CAD build for the part. Positions are in the model's coordinates, mm. Face numbers are marked on the shaded views. Coordinates: 2 decimals unless noted, no trailing zeros. Write each loop counter-clockwise with the first axis right and the second up, starting at its lowest first coordinate (ties: lowest second). Pieces come first, ordered by that corner, then holes.
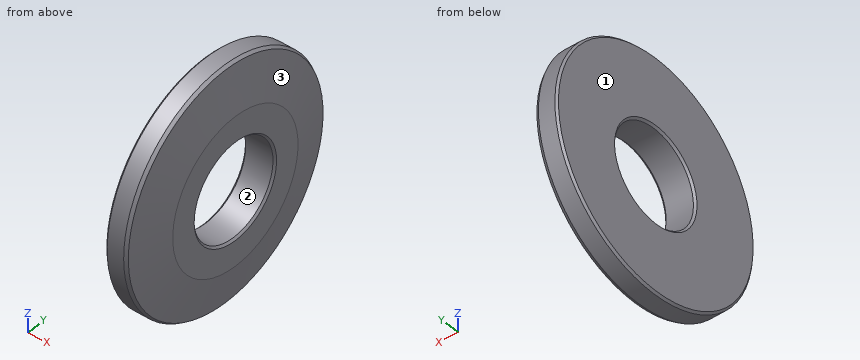
```python
from build123d import *

# Parameters (mm, degrees)
CHAMFER1_SIZE         = 0.25
CHAMFER1_EDGE_2_SIZE  = 0.25
CHAMFER1_EDGE_3_SIZE2 = 0.336401694
CHAMFER1_EDGE_3_SIZE  = 0.25
CHAMFER1_EDGE_4_SIZE  = 0.25


with BuildPart() as part:
    # Sketch1 → Revolve1 (revolve)
    with BuildSketch(Plane(origin=(0, 0, 0), x_dir=(1, 0, 0), z_dir=(0, 1, 0))):
        Polygon((2.7, 15), (4, 9.5), (4, 6), (0, 6), (0, 15), align=None)
    revolve(axis=Axis((0, 0, 0), (1, 0, 0)))

    # Chamfer1
    chamfer1_edges = [part.edges().sort_by_distance(p)[0] for p in [
        (0, 0, 6),
    ]]
    chamfer(chamfer1_edges, length=CHAMFER1_SIZE)

    # Chamfer1 edge 2
    chamfer1_edge_2_edges = [part.edges().sort_by_distance(p)[0] for p in [
        (4, 0, 6),
    ]]
    chamfer(chamfer1_edge_2_edges, length=CHAMFER1_EDGE_2_SIZE)

    # Chamfer1 edge 3
    chamfer1_edge_3_edges = [part.edges().sort_by_distance(p)[0] for p in [
        (2.7, 0, 15),
    ]]
    chamfer(chamfer1_edge_3_edges, length=CHAMFER1_EDGE_3_SIZE, length2=CHAMFER1_EDGE_3_SIZE2)

    # Chamfer1 edge 4
    chamfer1_edge_4_edges = [part.edges().sort_by_distance(p)[0] for p in [
        (0, 0, 15),
    ]]
    chamfer(chamfer1_edge_4_edges, length=CHAMFER1_EDGE_4_SIZE)


solid = part.part
```
Item 1: Saw through at A-A, the plane x = 1.35. Write the cut outline in (y, z), and give its area (3 significant figures).
Item 2: Two-plate mould, pull along Y, no slides. Class the marked faces 1, 2 and 3: +Y half, -Y half, draft (parallel to the pull), parting line (faces both ways), or undercut.
Item 3: Flat gauge pin, fed straight in: pin 1 Ø6 at (y, z) = (-7.5, -2) entering from -X. Where does the tip first touch, or does it go through?
Item 4: Saw through at B-B, the plane x = 3.1. Write the cut outline in (y, z), and give its area (3 significant figures).
Item 5: Wall check: line 1 along Y through (x, z) = (1.05, 0); line 2 along Z through (x, y) = (0.7, -3.5); line 3 along Z through (x, y) = (1.25, 5.5). Give the ranges that are in metal, low to high.
Working result:
1. outline: circle Ø30 at (0, 0); hole circle Ø12 at (0, 0)
1. area: 594 mm2
2. face 1: draft
2. face 2: undercut
2. face 3: parting line
3. pin 1: stops at x = 0
4. outline: circle Ø26.62 at (0, 0); hole circle Ø12 at (0, 0)
4. area: 443 mm2
5. line 1: y = -15 to -6, 6 to 15
5. line 2: z = -14.59 to -4.87, 4.87 to 14.59
5. line 3: z = -13.96 to -2.4, 2.4 to 13.96
